The model under review builds one solid part; all positions refer to its coordinate system, in mm. A direction names the side the tool comes from. Round coordinates to 2 decimals unless told otherwise and drop trailing zeros. Order: outer loops, then holes, each group sorted by start corner. A loop starts at its lowest first (then second) coordinate and runs counter-clockwise, first axis right, second up. Notation, with made-up numbers: M -25.75,13.5 L -5.75,13.5 A22 cw -5.75,32.5 Z; hole C 81,57.25 d11. An arc over 180 degrees is marked long. Use a Markdown table: item, result. Add a question column.
1. Consider section B-B on z = 70. State the section outline as (x, y) points, then the cut area to 3 significant figures.
2. Consider section D-D on y = 0. Count the separate pieces of the cut face and the enclosed holes in it, then the cut area to 3 significant figures.
3. The part is to be moulded in two halves that separate along Z. For faces 4 (the conical face through (418.5, 12, -2.7)), 5 (the flat face through (370, -53, 29)), 6 (the cylindrical face through (178.68, -50.59, 32.26)), say which applies: +Z half, -Z half, draft (parallel to the pull), parting line (faces both ways), or undercut.
4. Insertion check: P1, Ø11, axis at y = -58.5, z = 36.5, coming from the +X side; P2, Ø1, axis at x = 289.5, y = 36.5, coming from the +Z side; P3, Ø1, axis at y = -49.5, z = 52, coming from the -X side. Each pin has a flat end and moves straight along its axis. Give the tip position at first contact, or say it passes through.
5. For faces 1 (the flat face through (350, 58, -17)), 2 (the cylindrical face through (377.1, -50.59, 32.26)), 3 (the cylindrical face through (357.06, -64.72, -35.91)), list the 3-axis set-ups (+Z, -Z, +X, -X, +Y, -Y) from which the entire face can be reached by the end or side of a thin tool; tool diameter is ignored.
6. Consider section C-C on x = 294. State the section outline as (y, z) points, then the cut area to 3 significant figures.
7. Consider section A-A on z = 0. State the section outline as (x, y) points (1 decimal).
8. To check wall thickness, follow probe 1 along Y at (x, z) = (365.6, -35); probe 2 along X at (y, z) = (48.5, -47.5); probe 3 along Y at (x, z) = (349, -27). State the ranges of each line that lie inside material, in increasing order.
from build123d import *

# Parameters (mm, degrees)
CHAMFER1_SIZE                           = 2.5
CBORE_FOR_M8_HEX_HEAD_BOLT2_D           = 8.4
CBORE_FOR_M8_HEX_HEAD_BOLT2_CBORE_D     = 14
CBORE_FOR_M8_HEX_HEAD_BOLT2_CBORE_DEPTH = 5.68


with BuildPart() as part:
    # Sketch1 → Revolve1 (revolve)
    with BuildSketch(Plane(origin=(0, 0, 0), x_dir=(1, 0, 0), z_dir=(0, 1, 0)), mode=Mode.PRIVATE) as revolve1_sk:
        Polygon((0, 0), (0, 60), (350, 60), (350, 79), (370, 79), (370, 60), (384, 60), (435, 54), (443, 54), (443, 15.875), (394.6, 8.8165), (382.6, 8.8165), (382.6, 0), align=None)
    revolve(revolve1_sk.sketch.rotate(Axis((0, 0, 0), (1, 0, 0)), 180), axis=Axis((0, 0, 0), (1, 0, 0)))

    # Chamfer1
    chamfer1_edges = [part.edges().sort_by_distance(p)[0] for p in [
        (0, 0, -60),
    ]]
    chamfer(chamfer1_edges, length=CHAMFER1_SIZE)

    # CBORE for M8 Hex Head Bolt2 (through all)
    with Locations(Plane(origin=(370, 0, 0), x_dir=(0, 0, -1), z_dir=(1, 0, 0))):
        with Locations((-70, 0), (-35, 60.621778265), (35, 60.621778265), (70, 0), (35, -60.621778265), (-35, -60.621778265)):
            CounterBoreHole(CBORE_FOR_M8_HEX_HEAD_BOLT2_D / 2, CBORE_FOR_M8_HEX_HEAD_BOLT2_CBORE_D / 2, CBORE_FOR_M8_HEX_HEAD_BOLT2_CBORE_DEPTH)


solid = part.part
Answer block:
| question | item | result |
|---|---|---|
| 1 | outline | M 350,-36.62 L 370,-36.62 L 370,-7 L 364.32,-7 L 364.32,-4.2 L 350,-4.2 Z; M 350,4.2 L 364.32,4.2 L 364.32,7 L 370,7 L 370,36.62 L 350,36.62 Z |
| 1 | area | 1,260 mm^2 |
| 2 | separate pieces | 3 |
| 2 | enclosed holes | 0 |
| 2 | area | 51,700 mm^2 |
| 3 | face 4 | undercut |
| 3 | face 5 | draft |
| 3 | face 6 | parting line |
| 4 | P1 | x = 370 |
| 4 | P2 | z = 48 |
| 4 | P3 | x = 350 |
| 5 | face 1 | -X |
| 5 | face 2 | +X |
| 5 | face 3 | +X, -X |
| 6 | outline | C 0,0 d120 |
| 6 | area | 11,300 mm^2 |
| 7 | outline | M 0,-57.5 L 2.5,-60 L 350,-60 L 350,-79 L 370,-79 L 370,-60 L 384,-60 L 435,-54 L 443,-54 L 443,-15.9 L 394.6,-8.8 L 382.6,-8.8 L 382.6,8.8 L 394.6,8.8 L 443,15.9 L 443,54 L 435,54 L 384,60 L 370,60 L 370,79 L 350,79 L 350,60 L 2.5,60 L 0,57.5 Z |
| 8 | probe 1 | -70.82 to -67.62, -53.62 to 53.62, 67.62 to 70.82 |
| 8 | probe 2 | 350 to 370 |
| 8 | probe 3 | -53.58 to 53.58 |
